Source: CAD feature listing. Evaluate the final solid. Frame: model axes, mm. Face numbers are marked on the shaded views. A direction names the side the tool comes from. Round coordinates to 2 decimals unless told otherwise and drop trailing zeros. Loops run counter-clockwise (first coordinate to the right, second up) from the corner with the lowest first, then second, coordinate; pieces in that order, holes last.
(1) Section B-B, the plane x = -31.75. Return the cut outline in (y, z) (3 decimals).
(2) Mould query, pull axis X, two halves, no side actions, for the marked faces 3, 4 and 5. Classes: pulls with the +X half, pulls with the -X half, needs draft (parallel to the pull), parting line crosses it, or undercut.
(3) Section A-A, the plane z = 0. Return the cut outline in (x, y) (3 decimals).
(4) Set-up query: the marked faces 1 and 2. Return all of +Z, -Z, +X, -X, +Y, -Y with unobstructed straight access to the full face (end or side cutting, diameter ignored); none if empty.
(5) Material intervals for probe 1 along Z at (x, y) = (-31.75, -4.75) (3 decimals); probe 2 along X at (y, z) = (-4.5, -1); probe 3 along X at (y, z) = (-3.5, -6.5) (3 decimals), sorted ascending.
(6) Section C-C, the plane y = -6.75. Return the cut outline in (x, z) (3 decimals).
(7) First-contact query: pin 1 Ø3 at (x, y) = (39, -3) entering from -Z; pin 2 Ø5 at (x, y) = (0.5, -5.5) entering from +Z; pin 3 Ø5 at (x, z) = (4.99, -4.99) entering from -Y; pin 4 Ø7.5 at (x, z) = (-31.75, 0) entering from +Y. Flat tips, straight axial feed; report the tip coordinate or a pass-through.
```python
from build123d import *

# Parameters (mm, degrees)
F0_R     = 3.175
F1_DEPTH = 12.7
F2_R     = 1.27
F3_SIZE  = 0.635


with BuildPart() as f1:
    # F0 (on Front) → F1 (new body)
    with BuildSketch(Plane.XZ):
        with BuildLine():
            Line((-38.1, -19.05), (0, -19.05))
            Line((0, -19.05), (55.076783, -12.636062))
            ThreePointArc((55.076783, -12.636062), (61.089074, -9.508685), (63.5, -3.175))
            Line((63.5, -3.175), (63.5, 3.175))
            ThreePointArc((63.5, 3.175), (61.089074, 9.508685), (55.076783, 12.636062))
            Line((55.076783, 12.636062), (0, 19.05))
            Line((0, 19.05), (-38.1, 19.05))
            ThreePointArc((-38.1, 19.05), (-47.080256, 15.330256), (-50.8, 6.35))
            Line((-50.8, 6.35), (-50.8, -6.35))
            ThreePointArc((-50.8, -6.35), (-47.080256, -15.330256), (-38.1, -19.05))
        make_face()
        with Locations((-31.75, 0)):
            Circle(F0_R, mode=Mode.SUBTRACT)
        with BuildLine():
            ThreePointArc((4.9911, -3.0099), (6.39202, -6.39202), (3.0099, -4.9911))
            Line((3.0099, -4.9911), (-3.0099, -4.9911))
            ThreePointArc((-3.0099, -4.9911), (-6.39202, -6.39202), (-4.9911, -3.0099))
            Line((-4.9911, -3.0099), (-4.9911, 3.0099))
            ThreePointArc((-4.9911, 3.0099), (-6.39202, 6.39202), (-3.0099, 4.9911))
            Line((-3.0099, 4.9911), (3.0099, 4.9911))
            ThreePointArc((3.0099, 4.9911), (6.39202, 6.39202), (4.9911, 3.0099))
            Line((4.9911, 3.0099), (4.9911, -3.0099))
        make_face(mode=Mode.SUBTRACT)
    extrude(amount=F1_DEPTH)

    # F2
    f2_edges = [f1.edges().sort_by_distance(p)[0] for p in [
        (-19.05, -12.7, 19.05),
        (27.538392, -12.7, 15.843031),
        (-19.05, 0, 19.05),
        (27.538392, 0, 15.843031),
    ]]
    fillet(f2_edges, radius=F2_R)

    # F3
    f3_edges = [f1.edges().sort_by_distance(p)[0] for p in [
        (-34.925, -12.7, 0),
        (-4.9911, -12.7, 0),
        (0, -12.7, 4.9911),
        (4.9911, -12.7, 0),
        (0, -12.7, -4.9911),
        (6.39202, -12.7, -6.39202),
        (-6.39202, -12.7, -6.39202),
        (-6.39202, -12.7, 6.39202),
        (6.39202, -12.7, 6.39202),
        (-34.925, 0, 0),
        (-4.9911, 0, 0),
        (-6.39202, 0, 6.39202),
        (0, 0, 4.9911),
        (6.39202, 0, 6.39202),
        (4.9911, 0, 0),
        (6.39202, 0, -6.39202),
        (0, 0, -4.9911),
        (-6.39202, 0, -6.39202),
    ]]
    chamfer(f3_edges, length=F3_SIZE)


solid = f1.part
```
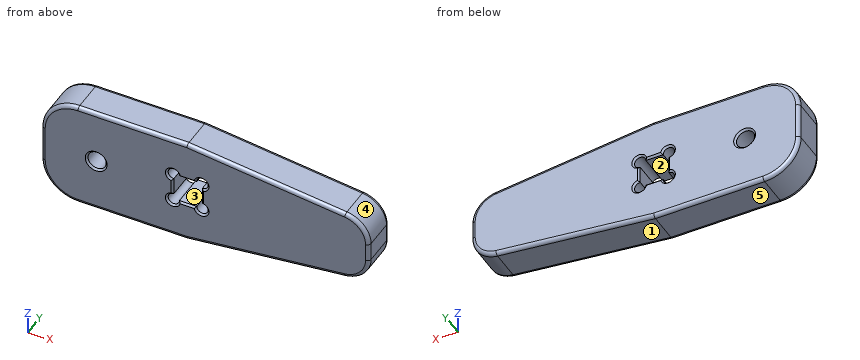
Output values:
1. outline: (-12.7, -17.78) arc R1.27 ccw to (-11.43, -19.05) - (-1.27, -19.05) arc R1.27 ccw to (0, -17.78) - (0, -3.81) - (-0.635, -3.175) - (-12.065, -3.175) - (-12.7, -3.81) - close; (-12.7, 3.81) - (-12.065, 3.175) - (-0.635, 3.175) - (0, 3.81) - (0, 17.78) arc R1.27 ccw to (-1.27, 19.05) - (-11.43, 19.05) arc R1.27 ccw to (-12.7, 17.78) - close
2. face 3: undercut
2. face 4: pulls with the +X half
2. face 5: needs draft
3. outline: (-50.8, -11.43) arc R1.27 ccw to (-49.53, -12.7) - (-35.56, -12.7) - (-34.925, -12.065) - (-34.925, -0.635) - (-35.56, 0) - (-49.53, 0) arc R1.27 ccw to (-50.8, -1.27) - close; (-28.575, -12.065) - (-27.94, -12.7) - (-5.626, -12.7) - (-4.991, -12.065) - (-4.991, -0.635) - (-5.626, 0) - (-27.94, 0) - (-28.575, -0.635) - close; (4.991, -12.065) - (5.626, -12.7) - (62.23, -12.7) arc R1.27 ccw to (63.5, -11.43) - (63.5, -1.27) arc R1.27 ccw to (62.23, 0) - (5.626, 0) - (4.991, -0.635) - close
4. face 1: -Z, +X, +Y, -Y
4. face 2: +Y, -Y
5. probe 1: z = -19.05 to -3.175, 3.175 to 19.05
5. probe 2: x = -50.8 to -34.76, -28.74 to -4.99, 4.99 to 63.5
5. probe 3: x = -50.799 to -6.275, -3.707 to 3.707, 6.275 to 62.901
6. outline: (-50.8, -6.35) arc R12.7 ccw to (-38.1, -19.05) - (0, -19.05) - (55.077, -12.636) arc R9.525 ccw to (63.5, -3.175) - (63.5, 3.175) arc R9.525 ccw to (55.077, 12.636) - (0, 19.05) - (-38.1, 19.05) arc R12.7 ccw to (-50.8, 6.35) - close; hole circle Ø6.35 at (-31.75, 0); hole (-4.991, -3.01) arc R1.981 ccw (long way) to (-3.01, -4.991) - (3.01, -4.991) arc R1.981 ccw (long way) to (4.991, -3.01) - (4.991, 3.01) arc R1.981 ccw (long way) to (3.01, 4.991) - (-3.01, 4.991) arc R1.981 ccw (long way) to (-4.991, 3.01) - close
7. pin 1: stops at z = -14.68
7. pin 2: stops at z = 19.05
7. pin 3: stops at y = -12.58
7. pin 4: stops at y = -0.06
